Source: CAD feature listing. Evaluate the final solid. Frame: model axes, mm. Face numbers are marked on the shaded views. A direction names the side the tool comes from. Coordinates: 2 decimals unless noted, no trailing zeros. Loops run counter-clockwise (first coordinate to the right, second up) from the corner with the lowest first, then second, coordinate; pieces in that order, holes last. Notation, with made-up numbers: (51, 19.25) -> (64, 19.25) arc R15 ccw to (64, 41.25) -> close; hole circle Ø3 at (14.25, 34.5). An arc over 180 degrees is marked (long way). One line per question, with ' | ' between items. Start each with the question number.
```python
from build123d import *

# Parameters (mm, degrees)
SKETCH1_W           = 42
SKETCH1_H           = 30
BOSS_EXTRUDE1_DEPTH = 2
SKETCH2_W           = 42
SKETCH2_H           = 30
SKETCH2_W_2         = 20.5
SKETCH2_H_2         = 2
SKETCH2_W_3         = 38
SKETCH2_H_3         = 22
BOSS_EXTRUDE2_DEPTH = 9
SKETCH6_W           = 2
SKETCH6_H           = 3
CUT_EXTRUDE2_DEPTH  = 2


with BuildPart() as part:
    # Sketch1 → Boss-Extrude1 (new body)
    with BuildSketch(Plane(origin=(0, 0, 0), x_dir=(1, 0, 0), z_dir=(0, 1, 0))):
        with Locations((21, 15)):
            Rectangle(SKETCH1_W, SKETCH1_H)
    extrude(amount=BOSS_EXTRUDE1_DEPTH)

    # Sketch2 → Boss-Extrude2 (add)
    with BuildSketch(Plane(origin=(0, 2, 0), x_dir=(1, 0, 0), z_dir=(0, 1, 0))):
        with Locations((21, 15)):
            Rectangle(SKETCH2_W, SKETCH2_H)
        with Locations((12.25, 27)):
            Rectangle(SKETCH2_W_2, SKETCH2_H_2, mode=Mode.SUBTRACT)
        with Locations((21, 13)):
            Rectangle(SKETCH2_W_3, SKETCH2_H_3, mode=Mode.SUBTRACT)
    extrude(amount=BOSS_EXTRUDE2_DEPTH)

    # Sketch6 → Cut-Extrude2 (cut)
    with BuildSketch(Plane.XY.offset(-24)):
        with Locations((4, 4.5)):
            Rectangle(SKETCH6_W, SKETCH6_H)
    extrude(amount=-CUT_EXTRUDE2_DEPTH, mode=Mode.SUBTRACT)


solid = part.part
```
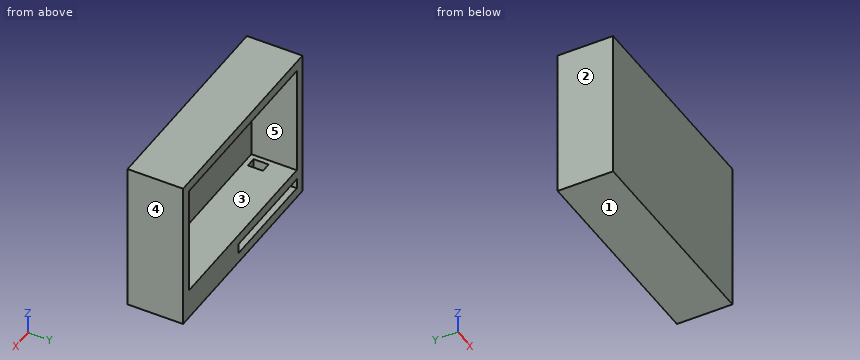
(1) Cut plane C-C, the plane z = -3.75. Return the cut outline in (x, y), and give its area (3 significant figures).
(2) Cut plane D-D, the plane x = 29.5. Return the cut outline in (y, z), and give its area (3 significant figures).
(3) Contact query for a flat-ended pin moving along its axis: pin 1 Ø3 at (x, z) = (20.5, -6) entering from +Y. Output: stop coordinate, or through.
(4) Access query for the marked faces 4 and 5. Directions: +Z, -Z, +X, -X, +Y, -Y. A direction counts if a zero-diameter tool reaches every point of the face in a straight line with its end or side. Return the directions, or none.
(5) Cut plane B-B, the plane x = 20. Return the cut outline in (y, z), and give its area (3 significant figures).
(6) Ray query, L1, parallel to Z at x = 16, y = 5.75; L2, parallel to X at y = 6.5, z = -16; L3, parallel to Z at x = 24, y = 8.25. Return the intervals inside material, ascending.
(7) Draft query along Z for the marked faces 1, 2 and 3. Return one class per face: pulls with the +Z half, pulls with the -Z half, needs draft (parallel to the pull), parting line crosses it, or undercut.
(8) Cut plane A-A, the plane y = 7. Return the cut outline in (x, z), and give its area (3 significant figures).
Here are the results:
1) outline: (0, 0) -> (42, 0) -> (42, 11) -> (40, 11) -> (40, 2) -> (2, 2) -> (2, 11) -> (0, 11) -> close | area: 120 mm2
2) outline: (0, -30) -> (11, -30) -> (11, -24) -> (2, -24) -> (2, -2) -> (11, -2) -> (11, 0) -> (0, 0) -> close | area: 132 mm2
3) pin 1: stops at y = 2
4) face 4: +Z, -Z, +X, +Y, -Y | face 5: +Y
5) outline: (0, -30) -> (11, -30) -> (11, -28) -> (2, -28) -> (2, -26) -> (11, -26) -> (11, -24) -> (2, -24) -> (2, -2) -> (11, -2) -> (11, 0) -> (0, 0) -> close | area: 114 mm2
6) L1: z = -30 to -28, -26 to -24, -2 to 0 | L2: x = 0 to 2, 40 to 42 | L3: z = -30 to -24, -2 to 0
7) face 1: pulls with the -Z half | face 2: needs draft | face 3: undercut
8) outline: (0, -30) -> (42, -30) -> (42, 0) -> (0, 0) -> close; hole (2, -28) -> (22.5, -28) -> (22.5, -26) -> (2, -26) -> close; hole (2, -24) -> (40, -24) -> (40, -2) -> (2, -2) -> close | area: 383 mm2
